Part model, mm, in its own coordinate system. A direction names the side the tool comes from. Give positions to 0.01 mm unless a question says otherwise; leave off trailing zeros. Order: outer loops, then holes, each group sorted by start corner. A loop starts at its lowest first (then second) coordinate and runs counter-clockwise, first axis right, second up. Notation, with made-up numbers: (74.25, -25) - (123.25, -25) arc R20 ccw to (123.25, -19) - close; hole circle Ø11 at (47.5, 83). An arc over 180 degrees is marked (long way). One line per item, written item: value.
```python
from build123d import *

# Parameters (mm, degrees)
F1_DEPTH = 1828.8
F3_DEPTH = 19.05
F5_DEPTH = 19.05


# Not quite as in the source:
# - the dataset's text gives a spline's control points without its knots; the knots are read off the source's solid


with BuildPart() as f1:
    # F0 (on Right) → F1 (new body)
    with BuildSketch(Plane.YZ):
        Polygon((-508, 0), (0, 0), (0, 304.8), (-19.05, 304.8), (-19.05, 19.05), (-508, 19.05), align=None)
    extrude(amount=F1_DEPTH)

    # F2 (on face) → F3 (join)
    with BuildSketch(Plane.YZ.offset(1828.8)):
        with BuildLine():
            Line((-508, 19.05), (-508, 0))
            Line((-508, 0), (0, 0))
            Line((0, 0), (0, 304.8))
            Line((0, 304.8), (-19.05, 304.8))
            Line((-19.05, 304.8), (-291.9989773071, 304.8))
            add(Edge.make_bspline(
                [(-291.9989773071, 304.8), (-492.9765110924, 298.0255581824), (-509.9911244928, 37.8132619011), (-507.4893097422, 43.3757593081), (-508, 19.05)],
                knots=[0, 0, 0, 0, 0.7436196079, 1, 1, 1, 1], degree=3))
        make_face()
    extrude(amount=-F3_DEPTH)

    # F4 (on face) → F5 (join)
    with BuildSketch(Plane(origin=(0, 0, 0), x_dir=(0, -1, 0), z_dir=(-1, 0, 0))):
        with BuildLine():
            Line((19.05, 304.8), (0, 304.8))
            Line((0, 304.8), (0, 0))
            Line((0, 0), (508, 0))
            Line((508, 0), (508, 19.05))
            add(Edge.make_bspline(
                [(291.9989773071, 304.8), (492.9765110924, 298.0255581824), (509.9911244928, 37.8132619011), (507.4893097422, 43.3757593081), (508, 19.05)],
                knots=[0, 0, 0, 0, 0.7436196079, 1, 1, 1, 1], degree=3))
            Line((291.9989773071, 304.8), (19.05, 304.8))
        make_face()
    extrude(amount=-F5_DEPTH)


solid = f1.part
```
1) Two-plate mould, pull along X, no slides. Class faces 3 (the face through (0, -259, 155)), 4 (the face through (902, -19.05, 164)), 5 (the face through (910, -16, 304.8)), 6 (the face through (1828.8, -259, 155)): pulls with the +X half, pulls with the -X half, needs draft (parallel to the pull), parting line crosses it, or undercut.
Answer:
face 3: pulls with the -X half
face 4: undercut
face 5: needs draft
face 6: pulls with the +X half
2) Wall check: line 1 along X through (y, z) = (-366.5, 87); line 2 along Z through (x, y) = (842.5, -263); line 3 along Y through (x, z) = (722.5, 175.5). Give the ranges that are in metal, low to high. Write a range as [from, to].
Answer:
line 1: x = [0, 19.05], [1809.75, 1828.8]
line 2: z = [0, 19.05]
line 3: y = [-19.05, 0]
3) Which spindle directions (+Z, -Z, +X, -X, +Y, -Y) get a long thin tool onto all of the face, cutting with end or side? Do faces 1 (the face through (902, 0, 150)), 2 (the face through (1809.75, -268, 164)). Say none if no direction does.
Answer:
face 1: +Z, -Z, +X, -X, +Y
face 2: +Z, -Y
4) Drop flat-ended pins along their axis: P1, Ø1.5, axis at x = 1361, y = -114.5, coming from the +Z side; P2, Ø5, axis at x = 1374, z = 249.5, coming from the -Y side. Give the stop position or say it passes through.
Answer:
P1: stops at z = 19.05
P2: stops at y = -19.05
5) Slice it at B-B on y = -160.5. Write the cut outline in (x, z).
Answer:
outline: (0, 0) - (1828.8, 0) - (1828.8, 304.8) - (1809.75, 304.8) - (1809.75, 19.05) - (19.05, 19.05) - (19.05, 304.8) - (0, 304.8) - close
6) Slice it at A-A on x = 1526. Write the cut outline in (y, z), then the cut area to 3 significant figures.
Answer:
outline: (-508, 0) - (0, 0) - (0, 304.8) - (-19.05, 304.8) - (-19.05, 19.05) - (-508, 19.05) - close
area: 15,100 mm2
